Could you check a few things on this model? Use its own coordinates, in mm. A direction names the side the tool comes from. Coordinates: 2 decimals unless noted, no trailing zeros. Loops run counter-clockwise (first coordinate to the right, second up) from the corner with the lowest first, then second, coordinate; pieces in that order, holes last. Notation, with made-up numbers: (76, 3.5) - (134, 3.5) arc R20 ccw to (134, 10.5) - close; hole circle Ø6 at (28.25, 59). An arc over 180 degrees is marked (long way). One line per item, written item: value. Start each with the question number.
(1) If we section it at D-D on y = 1.7: Write out the boundary of the cut face in (x, z), then the cut area to 3 significant figures.
(2) If we section it at B-B on x = 0: Write out the boundary of the cut face in (y, z).
(3) I'm going to push a flat-ended pin straight in: P1, Ø1, axis at x = 3, y = 1.5, coming from the +Z side. Where does the tip first touch, or does it pass through?
(4) If we section it at C-C on y = 3.6: Write out the boundary of the cut face in (x, z).
(5) If we mould it in two halves opening along Z, with no side actions, what happens to faces 3 (the face through (-0.07, 1.97, -10.27)), 4 (the face through (4.75, 2, 0)), 5 (the face through (-0.9, 1.97, -1.89))? For each: pulls with the +Z half, pulls with the -Z half, needs draft (parallel to the pull), parting line crosses it, or undercut.
(6) If we section it at A-A on z = -4.75: Write out the boundary of the cut face in (x, y).
(7) On a 3-axis mill with a long thin cutter (end or side, diameter ignored), from which of +Z, -Z, +X, -X, +Y, -Y can I reach the whole of each face in a straight line? I mean faces 1 (the face through (-4.076, 1.775, 5.465)), 2 (the face through (-4.75, 2, 0)). Say none if no direction works.
(8) If I drill on line 1 along Z through (x, y) = (1.75, 2); line 2 along Z through (x, y) = (-1.5, 1.15); line 3 along Y through (x, z) = (-4.3, 4.75), over which ranges is the centre line in solid material (lowest first)? Write a range as from..to.
Autodesk Inventor part; units mm, degrees
ref_plane "YZ Plane" through (0, 0, 0) normal (1, 0, 0) x (0, 1, 0)
ref_plane "XZ Plane" through (0, 0, 0) normal (0, 1, 0) x (-1, 0, 0)
ref_plane "XY Plane" through (0, 0, 0) normal (0, 0, 1) x (1, 0, 0)
sketch "Sketch1" plane through (0, 0, 0) normal (0, 1, 0) x (-1, 0, 0)
  line L0 (4.75, 9.5) -> (-4.75, 9.5)
  line L1 (-4.75, 9.5) -> (-4.75, -9.5)
  line L2 (-4.75, -9.5) -> (4.75, -9.5)
  line L3 (4.75, -9.5) -> (4.75, 9.5)
  line L4 (4.75, 9.5) -> (-4.75, -9.5) construction
  line L5 (-4.75, 9.5) -> (4.75, -9.5) construction
  arc A0 (-4.75, -9.5) -> (4.75, -9.5) centre (0, 4.7281) ccw
  arc A1 (4.75, 9.5) -> (-4.75, 9.5) centre (0, -4.7281) ccw
  point P0 (0, 0)
  dimension "d0" = 9.5
  dimension "d1" = 19
  dimension "d2" = 15
  dimension "d3" = 15
extrude "Extrusion1" add sketch "Sketch1" along normal blind 4
sketch "Sketch2" plane through (0, 4, 0) normal (0, 1, 0) x (1, 0, 0)
  arc A0 (4.75, 9.5) -> (-4.75, 9.5) centre (0, -4.7281) ccw
  point P0 (0, 0)
  point P1 (0, 4.75)
  point P2 (0, -4.75)
  dimension "d6" = 4.75
  dimension "d7" = 9.5
hole "Hole1" at (0, 4, -4.75) direction (0, -1, 0) diameter 6 end through all
hole "Hole2" at (0, 4, 4.75) at (0, 4, 4.7281) direction (0, -1, 0) diameter 7 end through all
sketch "Sketch3" plane through (-4.75, 0, -9.5) normal (-1, 0, 0) x (0, 0, 1)
  line L0 (19, 0) -> (19, 4)
  line L1 (0, 4) -> (19, 4)
  point P0 (9.5, 0)
  point P1 (14.25, 2)
  dimension "d22" = 4.75
  dimension "d23" = 2
hole "Hole3" at (-4.75, 2, 4.75) direction (1, 0, 0) diameter 1.5 depth 1.33 tip angle 118
properties material "Steel, Mild"
Values:
1. outline: (-4.75, -9.5) arc R15 ccw to (4.75, -9.5) - (4.75, 9.5) arc R15 ccw to (-4.75, 9.5) - (-4.75, 5.44) - (-3.43, 5.44) arc R3.5 cw to (3.5, 4.74) arc R3.5 cw to (-3.44, 4.06) - (-4.75, 4.06) - close; hole circle Ø6 at (0, -4.75)
1. area: 122 mm2
2. outline: (0, -10.27) - (4, -10.27) - (4, -7.75) - (0, -7.75) - close; (0, -1.75) - (4, -1.75) - (4, 1.23) - (0, 1.23) - close; (0, 8.25) - (4, 8.25) - (4, 10.27) - (0, 10.27) - close
3. P1: stops at z = 10.06
4. outline: (-4.75, -9.5) arc R15 ccw to (4.75, -9.5) - (4.75, 9.5) arc R15 ccw to (-4.75, 9.5) - close; hole (-3.5, 4.74) arc R3.5 ccw (long way) to (3.5, 4.74) arc R3.5 ccw (long way) to start; hole circle Ø6 at (0, -4.75)
5. face 3: pulls with the -Z half
5. face 4: needs draft
5. face 5: undercut
6. outline: (-4.75, 0) - (-3, 0) - (-3, 4) - (-4.75, 4) - close; (3, 0) - (4.75, 0) - (4.75, 4) - (3, 4) - close
7. face 1: -X
7. face 2: +Z, -Z, -X, +Y, -Y
8. line 1: z = -10.17..-7.19, -2.31..1.7, 7.78..10.17
8. line 2: z = -10.2..-7.35, -2.15..1.57, 7.91..10.2
8. line 3: y = 0..1.25, 2.75..4
